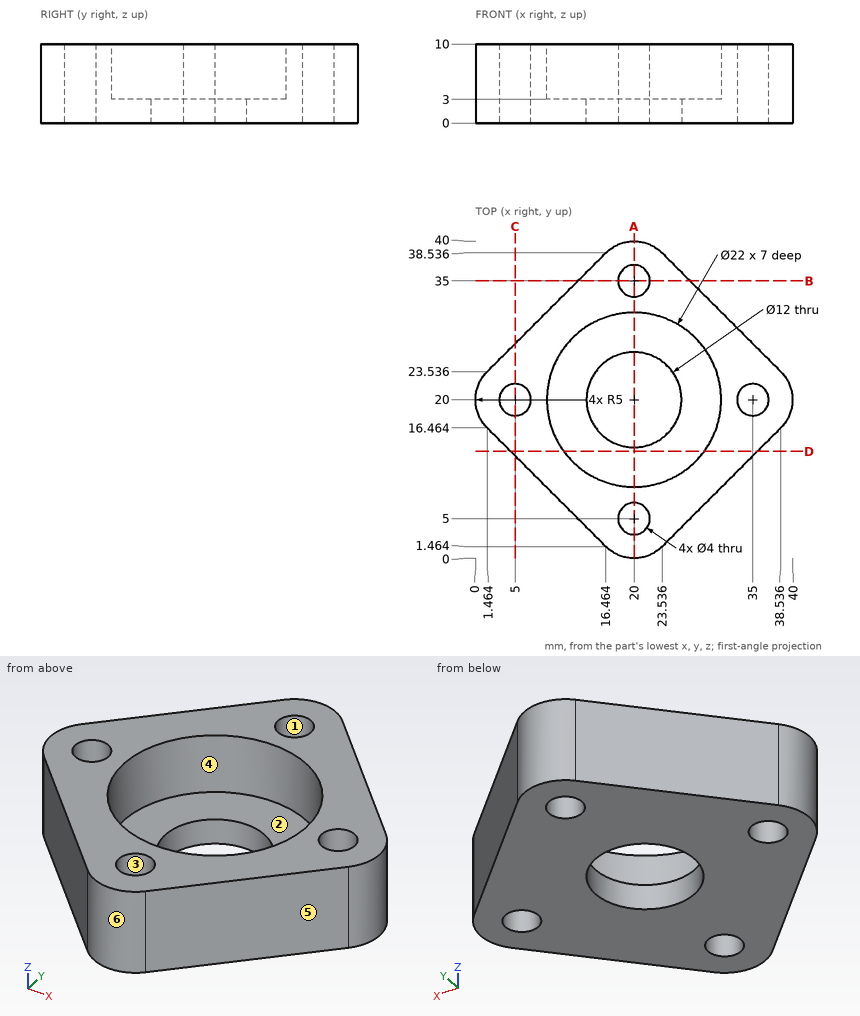
Input: dimensioned drawing with shaded views. Units: mm. Origin: part minimum x, y, z. A direction names the side the tool comes from. Give positions to 0.01 mm unless a question says otherwise; leave off trailing zeros. Write each loop counter-clockwise with the first axis right and the second up, starting at its lowest first coordinate (ties: lowest second). Pieces come first, ordered by that corner, then holes. Notation, with made-up numbers: M 1.25,62 L 30.25,62 A26 ccw 30.25,83 Z; hole C -14.5,-33 d10. An arc over 180 degrees is marked long. Return JSON: item names as keys, results as strings. Group by question number.
1) Cut plane D-D, the plane y = 13.5. Output: boundary loops of the cut face in (x, z) (1 decimal).
2) Set-up query: the marked faces 1 and 2. Return all of +Z, -Z, +X, -X, +Y, -Y with unobstructed straight access to the full face (end or side cutting, diameter ignored); none if empty.
3) Material intervals for line 1 along Y through (x, z) = (20, 6); line 2 along Y through (x, z) = (20, 1.1); line 3 along X through (y, z) = (18.5, 8.25) (1 decimal), sorted ascending. Write a range as [from, to].
4) Cut plane B-B, the plane y = 35. Output: boundary loops of the cut face in (x, z), plus the area to 3 significant figures.
5) Pull-direction query (X, two-part tool) for the marked faces 3, 4, 5 and 6; classes: pulls with the +X half, pulls with the -X half, needs draft (parallel to the pull), parting line crosses it, or undercut.
6) Pin query (flat end, axial travel): P1, Ø14, axis at x = 20, y = 20, coming from the +Z side; P2, Ø3, axis at y = 32, z = 4.5, coming from the -X side; P3, Ø3, axis at x = 10.5, z = 2, coming from the +Y side. Return the tip coordinate at first contact, or that it passes through.
7) Cut plane A-A, the plane x = 20. Output: boundary loops of the cut face in (y, z).
Recorded:
{
 "1": {"outline": "M 4.4,0 L 35.6,0 L 35.6,10 L 28.9,10 L 28.9,3 L 11.1,3 L 11.1,10 L 4.4,10 Z"},
 "2": {"face 1": "+Z, -Z", "face 2": "+Z"},
 "3": {"line 1": "y = [0, 3], [7, 9], [31, 33], [37, 40]", "line 2": "y = [0, 3], [7, 14], [26, 33], [37, 40]", "line 3": "x = [0.2, 3.7], [6.3, 9.1], [30.9, 33.7], [36.3, 39.8]"},
 "4": {"outline": "M 12.93,0 L 18,0 L 18,10 L 12.93,10 Z; M 22,0 L 27.07,0 L 27.07,10 L 22,10 Z", "area": "101 mm²"},
 "5": {"face 3": "undercut", "face 4": "undercut", "face 5": "pulls with the +X half", "face 6": "parting line crosses it"},
 "6": {"P1": "stops at z = 3", "P2": "stops at x = 8.43", "P3": "stops at y = 34.07"},
 "7": {"outline": "M 0,0 L 3,0 L 3,10 L 0,10 Z; M 7,0 L 14,0 L 14,3 L 9,3 L 9,10 L 7,10 Z; M 26,0 L 33,0 L 33,10 L 31,10 L 31,3 L 26,3 Z; M 37,0 L 40,0 L 40,10 L 37,10 Z"}
}
